Drawing for the job (mm, zero at the part's lowest x, y, z). Round coordinates to 2 decimals unless told otherwise and drop trailing zeros. Write each loop counter-clockwise with the first axis right and the second up, starting at its lowest first coordinate (ties: lowest second). Pieces come first, ordered by that corner, then holes. Notation, with made-up numbers: (80, 12.25) - (108, 12.25) arc R23 cw to (108, 28.25) - close; hole circle Ø8 at (-40, 44.5). An arc over 180 degrees is marked (long way). Answer in a Markdown table with one row per item.
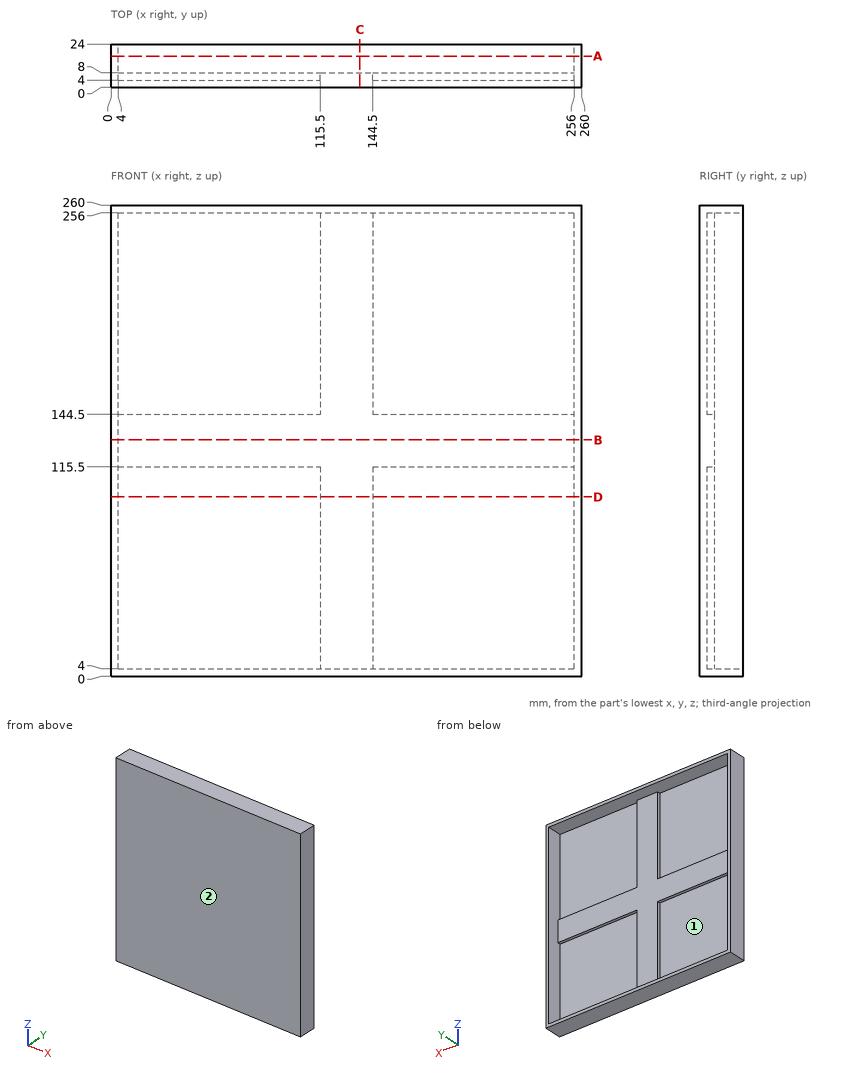
Q1. Saw through at D-D on z = 99. List the corners of the cut face in (x, y).
Computed:
| item | result |
|---|---|
| outline | (0, 0) - (260, 0) - (260, 24) - (256, 24) - (256, 4) - (144.5, 4) - (144.5, 8) - (115.5, 8) - (115.5, 4) - (4, 4) - (4, 24) - (0, 24) - close |
Q2. Pull direction Z, two halves, no side cores. Call the marked faces 1 and 2: released by +Z, released by -Z, zero draft, split by the parting line, or undercut.
Computed:
| item | result |
|---|---|
| face 1 | undercut |
| face 2 | zero draft |
Q3. Saw through at B-B on z = 130.5. List the corners of the cut face in (x, y).
Computed:
| item | result |
|---|---|
| outline | (0, 0) - (260, 0) - (260, 24) - (256, 24) - (256, 8) - (4, 8) - (4, 24) - (0, 24) - close |
Q4. Flat gauge pin, fed straight in: pin 1 (1.5 mm diameter, centred on x = 92.5, z = 136, fed in from +Y). Where does the tip first touch, or does it go through?
Computed:
| item | result |
|---|---|
| pin 1 | stops at y = 8 |
Q5. Saw through at A-A on y = 17.25. List the corners of the cut face in (x, z), then the cut area to 3 significant figures.
Computed:
| item | result |
|---|---|
| outline | (0, 0) - (260, 0) - (260, 260) - (0, 260) - close; hole (4, 4) - (256, 4) - (256, 256) - (4, 256) - close |
| area | 4,100 mm2 |
Q6. Drill centre lines: line 1 (X direction, y = 5.75, z = 194.5); line 2 (Z direction, x = 110, y = 12.75). Where is each one in solid material? Low to high.
Computed:
| item | result |
|---|---|
| line 1 | x = 0 to 4, 115.5 to 144.5, 256 to 260 |
| line 2 | z = 0 to 4, 256 to 260 |
Q7. Saw through at C-C on x = 137.5. List the corners of the cut face in (y, z).
Computed:
| item | result |
|---|---|
| outline | (0, 0) - (24, 0) - (24, 4) - (8, 4) - (8, 256) - (24, 256) - (24, 260) - (0, 260) - close |
